Build history of the part. All positions in model axes, mm. A direction names the side the tool comes from. Round coordinates to 2 decimals unless told otherwise and drop trailing zeros. Loops run counter-clockwise (first coordinate to the right, second up) from the corner with the lowest first, then second, coordinate; pieces in that order, holes last. Notation, with made-up numbers: M -14,-15 L -10,-15 A16 cw -10,-2 Z; hole C -4,23.5 d8. An arc over 180 degrees is marked long. Use one line per item in the form item = value. Start each with the question number.
```python
from build123d import *

# Parameters (mm, degrees)
SKETCH1_W           = 68
SKETCH1_H           = 68
BOSS_EXTRUDE1_DEPTH = 10
BOSS_EXTRUDE2_DEPTH = 3
BOSS_EXTRUDE3_DEPTH = 7
BOSS_EXTRUDE4_START = 3
BOSS_EXTRUDE4_DEPTH = 3
BOSS_EXTRUDE5_START = 7
BOSS_EXTRUDE5_DEPTH = 7
SKETCH6_W           = 42.5
SKETCH6_H           = 42.5
CUT_EXTRUDE1_DEPTH  = 3
SKETCH8_R           = 1.5
CUT_EXTRUDE2_DEPTH  = 5
SKETCH9_W           = 4
SKETCH9_H           = 7
BOSS_EXTRUDE6_DEPTH = 6
SKETCH10_R          = 1.5
CUT_EXTRUDE3_DEPTH  = 10
SKETCH11_R          = 1
CUT_EXTRUDE4_DEPTH  = 20
SKETCH13_W          = 7
SKETCH13_H          = 16
BOSS_EXTRUDE7_DEPTH = 12
CUT_EXTRUDE5_DEPTH  = 10
BOSS_EXTRUDE8_START = -7
BOSS_EXTRUDE8_DEPTH = 7


with BuildPart() as part:
    # Sketch1 → Boss-Extrude1 (new body)
    with BuildSketch(Plane.XY):
        with Locations((-34, -34)):
            Rectangle(SKETCH1_W, SKETCH1_H)
    extrude(amount=BOSS_EXTRUDE1_DEPTH)

    # Sketch2 → Boss-Extrude2 (add)
    with BuildSketch(Plane.ZY.offset(68)):
        with BuildLine():
            Line((10, -19.354101966), (10, -12.645898034))
            ThreePointArc((10, -12.645898034), (5.5, -16), (10, -19.354101966))
        make_face()
        with BuildLine():
            Line((10, -55.354101966), (10, -48.645898034))
            ThreePointArc((10, -48.645898034), (5.5, -52), (10, -55.354101966))
        make_face()
    extrude(amount=BOSS_EXTRUDE2_DEPTH)

    # Sketch3 → Boss-Extrude3 (add)
    with BuildSketch(Plane.ZY.offset(71)):
        with BuildLine():
            ThreePointArc((10, -49.984435563), (6.75, -52), (10, -54.015564437))
            Line((10, -54.015564437), (10, -49.984435563))
        make_face()
        with BuildLine():
            ThreePointArc((10, -13.984435563), (6.75, -16), (10, -18.015564437))
            Line((10, -18.015564437), (10, -13.984435563))
        make_face()
    extrude(amount=BOSS_EXTRUDE3_DEPTH)

    # Sketch4 → Boss-Extrude4 (add)
    with BuildSketch(Plane(origin=(0, 0, 0), x_dir=(0, 0, -1), z_dir=(1, 0, 0)).offset(BOSS_EXTRUDE4_START)):
        with BuildLine():
            ThreePointArc((-5.5, -16), (-6.908349934, -13.19375696), (-10, -12.645898034))
            Line((-10, -12.645898034), (-10, -19.354101966))
            ThreePointArc((-10, -19.354101966), (-6.908349934, -18.80624304), (-5.5, -16))
        make_face()
        with BuildLine():
            ThreePointArc((-5.5, -52), (-6.908349934, -49.19375696), (-10, -48.645898034))
            Line((-10, -48.645898034), (-10, -55.354101966))
            ThreePointArc((-10, -55.354101966), (-6.908349934, -54.80624304), (-5.5, -52))
        make_face()
    extrude(amount=-BOSS_EXTRUDE4_DEPTH)

    # Sketch5 → Boss-Extrude5 (add)
    with BuildSketch(Plane(origin=(3, 0, 0), x_dir=(0, 0, -1), z_dir=(1, 0, 0)).offset(BOSS_EXTRUDE5_START)):
        with BuildLine():
            ThreePointArc((-6.75, -16), (-7.814145877, -14.087867682), (-10, -13.984435563))
            Line((-10, -13.984435563), (-10, -18.015564437))
            ThreePointArc((-10, -18.015564437), (-7.814145877, -17.912132318), (-6.75, -16))
        make_face()
        with BuildLine():
            ThreePointArc((-6.75, -52), (-7.814145877, -50.087867682), (-10, -49.984435563))
            Line((-10, -49.984435563), (-10, -54.015564437))
            ThreePointArc((-10, -54.015564437), (-7.814145877, -53.912132318), (-6.75, -52))
        make_face()
    extrude(amount=-BOSS_EXTRUDE5_DEPTH)

    # Sketch6 → Cut-Extrude1 (cut)
    with BuildSketch(Plane(origin=(0, 0, 0), x_dir=(-1, 0, 0), z_dir=(0, 0, -1))):
        with Locations((34, -34)):
            Rectangle(SKETCH6_W, SKETCH6_H)
    extrude(amount=-CUT_EXTRUDE1_DEPTH, mode=Mode.SUBTRACT)

    # Sketch8 → Cut-Extrude2 (cut)
    with BuildSketch(Plane(origin=(0, 0, 0), x_dir=(-1, 0, 0), z_dir=(0, 0, -1))):
        with Locations((20.75, -7.75)):
            Circle(SKETCH8_R)
        with Locations(Location((47.25, -7.75, 0), (0, 0, 180))):
            Circle(SKETCH8_R)
        with Locations((47.25, -60.25)):
            Circle(SKETCH8_R)
        with Locations(Location((20.75, -60.25, 0), (0, 0, 180))):
            Circle(SKETCH8_R)
    extrude(amount=-CUT_EXTRUDE2_DEPTH, mode=Mode.SUBTRACT)

    # Sketch9 → Boss-Extrude6 (add)
    with BuildSketch(Plane(origin=(0, 0, 0), x_dir=(-1, 0, 0), z_dir=(0, 0, -1))):
        with Locations((2, -27.5)):
            Rectangle(SKETCH9_W, SKETCH9_H)
        with Locations((2, -40.5)):
            Rectangle(SKETCH9_W, SKETCH9_H)
    extrude(amount=BOSS_EXTRUDE6_DEPTH)

    # Sketch10 → Cut-Extrude3 (cut)
    with BuildSketch(Plane(origin=(0, 0, 0), x_dir=(-1, 0, 0), z_dir=(0, 0, -1))):
        with Locations((7.75, -27.5)):
            Circle(SKETCH10_R)
        with Locations(Location((7.75, -40.5, 0), (0, 0, 180))):
            Circle(SKETCH10_R)
    extrude(amount=-CUT_EXTRUDE3_DEPTH, mode=Mode.SUBTRACT)

    # Sketch11 → Cut-Extrude4 (cut)
    with BuildSketch(Plane.XY.offset(10)):
        with Locations((-62, -52)):
            Circle(SKETCH11_R)
        with Locations(Location((-62, -16, 0), (0, 0, 180))):
            Circle(SKETCH11_R)
        with Locations(Location((-6, -52, 0), (0, 0, 180))):
            Circle(SKETCH11_R)
        with Locations((-6, -16)):
            Circle(SKETCH11_R)
    extrude(amount=-CUT_EXTRUDE4_DEPTH, mode=Mode.SUBTRACT)

    # Sketch13 → Boss-Extrude7 (add)
    with BuildSketch(Plane(origin=(0, 0, 0), x_dir=(-1, 0, 0), z_dir=(0, 0, -1))):
        with Locations((62, -34)):
            Rectangle(SKETCH13_W, SKETCH13_H)
    extrude(amount=BOSS_EXTRUDE7_DEPTH)

    # Sketch15 → Cut-Extrude5 (cut)
    with BuildSketch(Plane.ZY.offset(65.5)):
        Polygon((-12, -32), (-3, -32), (-5, -30), (-12, -30), align=None)
        Polygon((-12, -38), (-12, -36), (-3, -36), (-5, -38), align=None)
    extrude(amount=-CUT_EXTRUDE5_DEPTH, mode=Mode.SUBTRACT)

    # Sketch16 → Boss-Extrude8 (add)
    with BuildSketch(Plane.ZY.offset(65.5).offset(BOSS_EXTRUDE8_START)):
        Polygon((0, -26), (-12, -26), (0, -21), align=None)
        Polygon((-12, -42), (0, -47), (0, -42), align=None)
    extrude(amount=BOSS_EXTRUDE8_DEPTH)


solid = part.part
```
Q1. Saw through at A-A (y = -27.5). Give the cut face in (x, z), and give its area (4 significant figures).
Q2. Saw through at C-C (z = -8). Give the cut face in (x, y), and give its area (3 significant figures).
Q3. Tool access for faces 1 (the face through (-2, -31, -3)), 2 (the face through (-74.45, -51.94, 6.75)), 3 (the face through (-55.25, -34, 1)), 4 (the face through (-62, -36, -8)): list every direction of +Z, -Z, +X, -X, +Y, -Y with a clear straight run to the whole face (end or side of a thin tool).
Q4. Wall check: probe 1 along Y at (x, z) = (-62, 6); probe 2 along Y at (x, z) = (-47.25, 2.35); probe 3 along Y at (x, z) = (-7.75, 2.5). Give the ranges that are in metal, low to high.
Q5. Saw through at B-B (x = -23.5). Give the cut face in (y, z).
Q6. Saw through at D-D (y = -35). Give the cut face in (x, z), and give its area (4 significant figures).
Q7. Drop flat-ended pins along their axis: P1, Ø3.5, axis at y = -29.5, z = -8.5, coming from the -X side; P2, Ø5.5, axis at x = -60.5, z = -10, coming from the -Y side; P3, Ø1.5, axis at x = -20.5, y = -60, coming from the -Z side. Give the stop position or say it passes through.
Q8. Pull direction X, two halves, no side cores. Call faces 5 (the face through (-71, -52.7, 6.7)), 6 (the face through (-34, -55.25, 1)), 7 (the face through (-2, -44, -3)): pulls with the +X half, pulls with the -X half, needs draft (parallel to the pull), parting line crosses it, or undercut.
Filled in:
q1.outline = M -68,0 L -65.5,0 L -65.5,-12 L -58.5,-12 L -58.5,0 L -55.25,0 L -55.25,3 L -12.75,3 L -12.75,0 L -9.25,0 L -9.25,10 L -68,10 Z; M -6.25,0 L -4,0 L -4,-6 L 0,-6 L 0,10 L -6.25,10 Z
q1.area = 630.5 mm²
q2.outline = M -65.5,-43.67 L -58.5,-43.67 L -58.5,-38 L -65.5,-38 Z; M -65.5,-36 L -58.5,-36 L -58.5,-32 L -65.5,-32 Z; M -65.5,-30 L -58.5,-30 L -58.5,-24.33 L -65.5,-24.33 Z
q2.area = 107 mm²
q3.face_1 = -Z, +X
q3.face_2 = -X
q3.face_3 = -Z
q3.face_4 = -Z, +X, -X
q4.probe_1 = -68 to -53, -51 to -17, -15 to 0
q4.probe_2 = -68 to -61.75, -58.75 to -55.25, -12.75 to -9.25, -6.25 to 0
q4.probe_3 = -68 to -42, -39 to -29, -26 to 0
q5.outline = M -68,0 L -55.25,0 L -55.25,3 L -12.75,3 L -12.75,0 L 0,0 L 0,10 L -68,10 Z
q6.outline = M -68,0 L -65.5,0 L -65.5,-12 L -58.5,-12 L -58.5,0 L -55.25,0 L -55.25,3 L -12.75,3 L -12.75,0 L 0,0 L 0,10 L -68,10 Z
q6.area = 636.5 mm²
q7.P1 = -65.5
q7.P2 = -43.98
q7.P3 = 5
q8.face_5 = pulls with the -X half
q8.face_6 = undercut
q8.face_7 = needs draft
